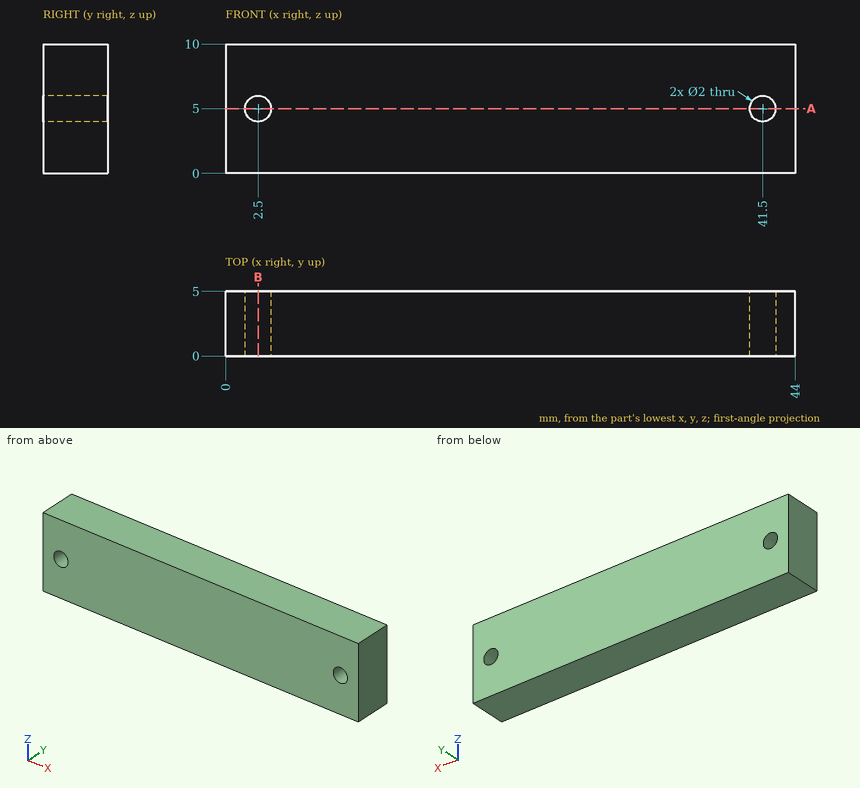
The figure shows three views and two pictorial views of one solid part (mm, origin at its lowest corner). Answer the questions. Give positions to 0.01 mm unless a question says otherwise; leave off trailing zeros. Loops run counter-clockwise (first coordinate to the right, second up) from the corner with the lowest first, then second, coordinate; pieces in that order, holes last. Notation, with made-up numbers: (6.5, 23) -> (22.5, 23) arc R8 ccw to (22.5, 29) -> close; hole circle Ø8 at (73.5, 84). An arc over 180 degrees is marked (long way). Put each result on its own line as item: value. Start each with the question number.
Item 1: The part is cut by section A-A (z = 5). Give the vertices of the cut face in (x, y).
Item 2: This flat-tipped pin is pushed along its axis until it touches: P1, Ø3, axis at y = 3.5, z = 8.5, coming from the -X side. Where does it stop, or does it pass through?
Item 3: The part is cut by section B-B (x = 2.5). Give the vertices of the cut face in (y, z), then the cut area to 3 significant figures.
Item 4: Find the intervals of material crossed by L1, parallel to Z at x = 41.5, y = 3.95, in increasing order. Write a range as [from, to].
Answers below:
1. outline: (0, 0) -> (1.5, 0) -> (1.5, 5) -> (0, 5) -> close; (3.5, 0) -> (40.5, 0) -> (40.5, 5) -> (3.5, 5) -> close; (42.5, 0) -> (44, 0) -> (44, 5) -> (42.5, 5) -> close
2. P1: x = 0
3. outline: (0, 0) -> (5, 0) -> (5, 4) -> (0, 4) -> close; (0, 6) -> (5, 6) -> (5, 10) -> (0, 10) -> close
3. area: 40.0 mm2
4. L1: [0, 4], [6, 10]
